Source: CAD feature listing. Evaluate the final solid. Frame: model axes, mm. A direction names the side the tool comes from. Give positions to 0.01 mm unless a question says otherwise; leave off trailing zeros. Loops run counter-clockwise (first coordinate to the right, second up) from the corner with the lowest first, then second, coordinate; pieces in that order, holes last. Notation, with made-up numbers: M 35,52 L 81,52 A22 ccw 81,78 Z; hole C 15.5,76 d11. An arc over 180 degrees is marked long. Answer in a Markdown table with one row per item.
```python
from build123d import *

# Parameters (mm, degrees)
F1_DEPTH = 25.4
F3_DEPTH = 50.8


with BuildPart() as f1:
    # F0 (on Front) → F1 (new body)
    with BuildSketch(Plane.XZ):
        with BuildLine():
            ThreePointArc((12.7, 25.4), (0, 38.1), (-12.7, 25.4))
            Line((-12.7, 25.4), (-12.7, -25.4))
            Line((-12.7, -25.4), (-9.525, -25.4))
            Line((-9.525, -25.4), (-9.525, 25.4))
            ThreePointArc((-9.525, 25.4), (0, 34.925), (9.525, 25.4))
            Line((9.525, 25.4), (9.525, -25.4))
            Line((9.525, -25.4), (12.7, -25.4))
            Line((12.7, -25.4), (12.7, 25.4))
        make_face()
    extrude(amount=F1_DEPTH)

    # F2 (on face) → F3 (cut, symmetric)
    with BuildSketch(Plane(origin=(-12.7, 0, 0), x_dir=(0, -1, 0), z_dir=(-1, 0, 0))):
        with BuildLine():
            ThreePointArc((15.875, -19.05), (10.454936, -16.804936), (12.7, -22.225))
            ThreePointArc((12.7, -22.225), (14.945064, -21.295064), (15.875, -19.05))
        make_face()
    extrude(amount=F3_DEPTH, both=True, mode=Mode.SUBTRACT)


solid = f1.part
```
Q1. Mould query, pull axis X, two halves, no side actions, for faces 1 (the flat face through (12.7, -13, 0)), 2 (the cylindrical face through (0.279, -12.522, 38.097)), 3 (the flat face through (-9.525, -13, 0)), 4 (the cylindrical face through (-0.209, -12.522, 34.923)). Classes: +X half, -X half, draft (parallel to the pull), parting line (faces both ways), or undercut.
Values follow:
| item | result |
|---|---|
| face 1 | +X half |
| face 2 | parting line |
| face 3 | undercut |
| face 4 | undercut |
Q2. Section query D-D (x = -4.75). Output: boundary loops of the cut face in (y, z), plus the area to 3 significant figures.
Values follow:
| item | result |
|---|---|
| outline | M -25.4,33.66 L 0,33.66 L 0,37.18 L -25.4,37.18 Z |
| area | 89.5 mm^2 |
Q3. Section query A-A (z = 20.5). Output: boundary loops of the cut face in (x, y) (3 decimals), plus the area to 3 significant figures.
Values follow:
| item | result |
|---|---|
| outline | M -12.7,-25.4 L -9.525,-25.4 L -9.525,0 L -12.7,0 Z; M 9.525,-25.4 L 12.7,-25.4 L 12.7,0 L 9.525,0 Z |
| area | 161 mm^2 |
Q4. Contact query for a flat-ended pin moving along its axis: pin 1 Ø10 at (x, z) = (-3.5, -5.5) entering from -Y. Output: stop coordinate, or through.
Values follow:
| item | result |
|---|---|
| pin 1 | through |
Q5. Section query B-B (y = -1.25). Output: boundary loops of the cut face in (x, z) (3 decimals), plus the area to 3 significant figures.
Values follow:
| item | result |
|---|---|
| outline | M -12.7,-25.4 L -9.525,-25.4 L -9.525,25.4 A9.525 cw 9.525,25.4 L 9.525,-25.4 L 12.7,-25.4 L 12.7,25.4 A12.7 ccw -12.7,25.4 Z |
| area | 433 mm^2 |
Q6. Reachability of faces 5 (the flat face through (11, -13, -25.4)), 6 (the flat face through (9.525, -13, 0)) from +Z, -Z, +X, -X, +Y, -Y: full face, straight path, thin tool, end or side. Return the list, or none.
Values follow:
| item | result |
|---|---|
| face 5 | -Z, +X, -X, +Y, -Y |
| face 6 | -Z, +Y, -Y |
Q7. Ray query, probe 1 along Y at (x, z) = (11.3, -19.05) (3 decimals); probe 2 along X at (y, z) = (-10, -5.5) (3 decimals); probe 3 along Z at (x, y) = (10.4, -12.7) (3 decimals). Return the intervals inside material, ascending. Write a range as from..to.
Values follow:
| item | result |
|---|---|
| probe 1 | -25.4..-15.875, -9.525..0 |
| probe 2 | -12.7..-9.525, 9.525..12.7 |
| probe 3 | -25.4..-22.225, -15.875..32.689 |
Q8. Section query C-C (x = 0). Output: boundary loops of the cut face in (y, z) (3 decimals).
Values follow:
| item | result |
|---|---|
| outline | M -25.4,34.925 L 0,34.925 L 0,38.1 L -25.4,38.1 Z |
